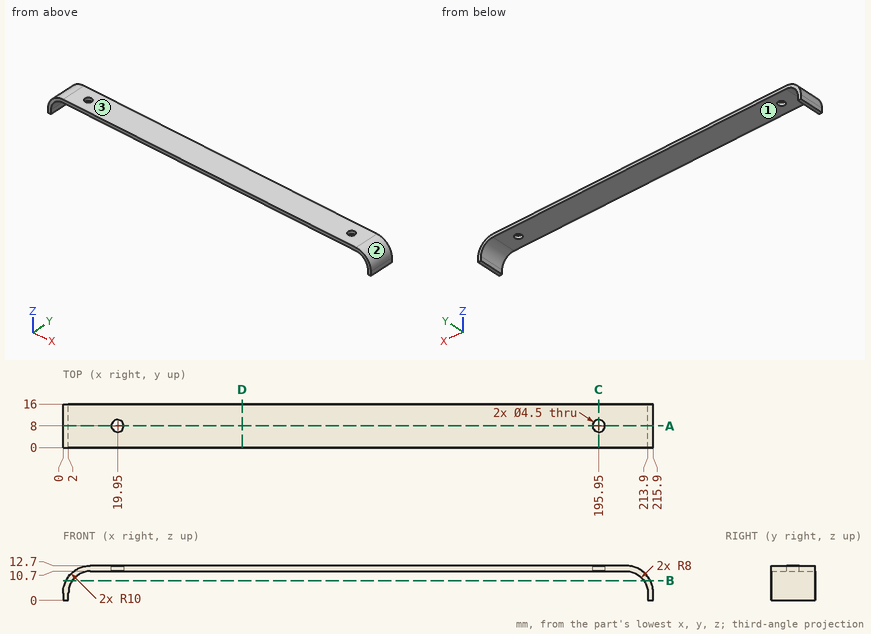
Here's the drawing with two shaded views (mm, measured from the low corner). I have some questions. Coordinates: 2 decimals unless noted, no trailing zeros. Loops run counter-clockwise (first coordinate to the right, second up) from the corner with the lowest first, then second, coordinate; pieces in that order, holes last.
Item 1: Suppose I cut it at A-A (y = 8). Please give me the cut outline in (x, z), then the cut area to 3 significant figures.
Answers below:
outline: (0, 0) - (2, 0) - (2, 2.7) arc R8 cw to (10, 10.7) - (17.7, 10.7) - (17.7, 12.7) - (10, 12.7) arc R10 ccw to (0, 2.7) - close; (22.2, 10.7) - (193.7, 10.7) - (193.7, 12.7) - (22.2, 12.7) - close; (198.2, 10.7) - (205.9, 10.7) arc R8 cw to (213.9, 2.7) - (213.9, 0) - (215.9, 0) - (215.9, 2.7) arc R10 ccw to (205.9, 12.7) - (198.2, 12.7) - close
area: 441 mm2
Item 2: Suppose I cut it at D-D (x = 65.5). Please give me the cut outline in (y, z), then the cut area to 3 significant figures.
Answers below:
outline: (0, 10.7) - (16, 10.7) - (16, 12.7) - (0, 12.7) - close
area: 32.0 mm2
Item 3: Please list where these lines run through material, in increasing order: L1, parallel to X at y = 15.25, z = 3.5; L2, parallel to Y at x = 195.95, z = 11.15; L3, parallel to Z at x = 188.5, y = 12.25.
Answers below:
L1: x = 0.03 to 2.04, 213.86 to 215.87
L2: y = 0 to 5.75, 10.25 to 16
L3: z = 10.7 to 12.7
Item 4: If we mould it in two halves opening along X, with no side actions, what happens to the marked faces 1, 2 and 3? For each: released by +X, released by -X, zero draft, split by the parting line, or undercut.
Answers below:
face 1: undercut
face 2: released by +X
face 3: zero draft
Item 5: Suppose I cut it at B-B (z = 7.25). Please give me the cut outline in (x, y).
Answers below:
outline: (1.1, 0) - (3.42, 0) - (3.42, 16) - (1.1, 16) - close; (212.48, 0) - (214.8, 0) - (214.8, 16) - (212.48, 16) - close
Item 6: Suppose I cut it at C-C (x = 195.95). Please give me the cut outline in (y, z), then the cut area to 3 significant figures.
Answers below:
outline: (0, 10.7) - (5.75, 10.7) - (5.75, 12.7) - (0, 12.7) - close; (10.25, 10.7) - (16, 10.7) - (16, 12.7) - (10.25, 12.7) - close
area: 23.0 mm2
Item 7: I'm going to push flat-ended pins straight in: pin 1 (4 mm diameter, centred on x = 195.95, y = 8, fed in from +Z); pin 2 (3 mm diameter, centred on x = 149.5, y = 11, fed in from -Z); pin 3 (1 mm diameter, centred on y = 5.5, z = 3.5, fed in from -X). Where does each tip first touch, or does it pass through?
Answers below:
pin 1: passes through
pin 2: stops at z = 10.7
pin 3: stops at x = 0
